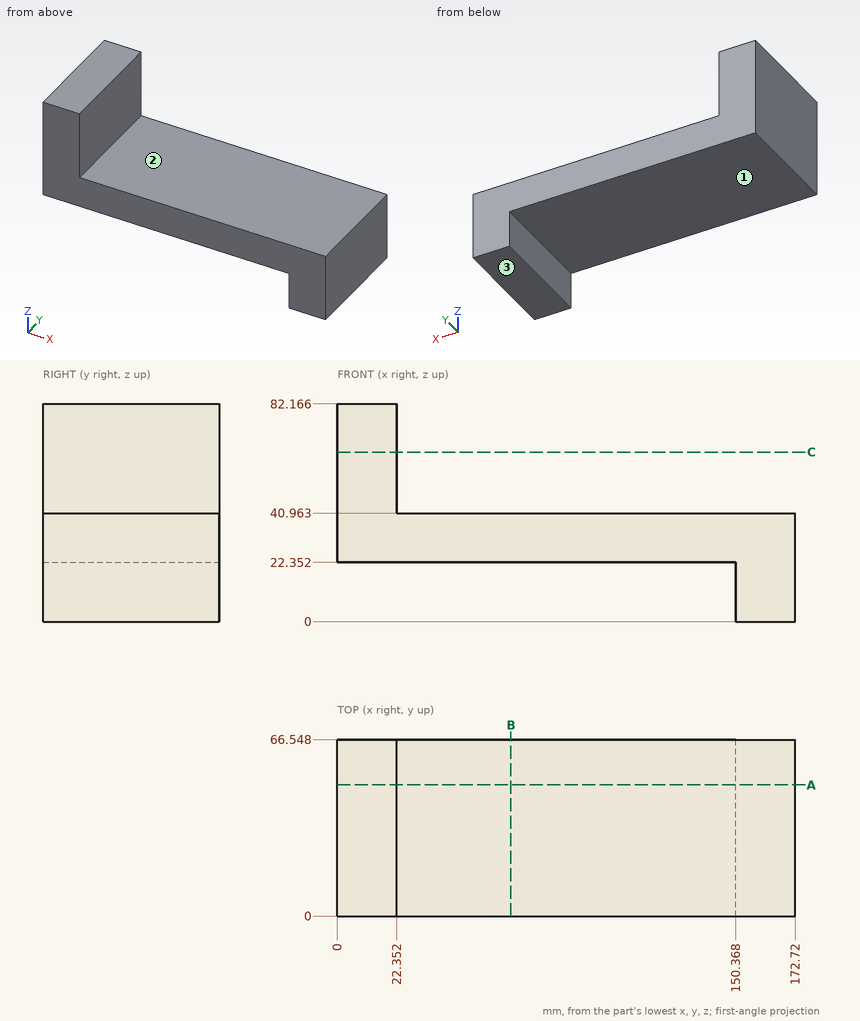
Verification items for this drawing (mm, ordinates from the low corner). A direction names the side the tool comes from. Coordinates: 2 decimals unless noted, no trailing zeros. Write each loop counter-clockwise with the first axis right and the second up, starting at its lowest first coordinate (ties: lowest second). Pieces come first, ordered by that corner, then holes. Notation, with made-up numbers: M 21.5,-36.5 L 72.5,-36.5 A4 cw 72.5,-31.5 Z; hole C 84.25,-34 d11. An arc over 180 degrees is marked long. Use CSV: the item, a comma, the result in double quotes.
Q1. Thickness scan on line 1 along Z through (x, y) = (90.5, 59); line 2 along X through (y, z) = (62, 21.5); line 3 along X through (y, z) = (21.5, 61). Record the ranges inside material, lowest first. Write a range as [from, to].
Computed values:
line 1,"[22.35, 40.96]"
line 2,"[150.37, 172.72]"
line 3,"[0, 22.35]"
Q2. Section check A-A, the plane y = 49.5. Enter the section's corners in (x, z) (1 decimal).
Computed values:
outline,"M 0,22.4 L 150.4,22.4 L 150.4,0 L 172.7,0 L 172.7,41 L 22.4,41 L 22.4,82.2 L 0,82.2 Z"
Q3. Set-up check for the marked faces 1, 2 and 3: record each of +Z, -Z, +X, -X, +Y, -Y from which the full face is reachable in a straight line by a thin tool's end or side.
Computed values:
face 1,"-Z, -X, +Y, -Y"
face 2,"+Z, +X, +Y, -Y"
face 3,"-Z, +X, -X, +Y, -Y"
Q4. Section check C-C, the plane z = 64. Enter the section's corners in (x, y).
Computed values:
outline,"M 0,0 L 22.35,0 L 22.35,66.55 L 0,66.55 Z"
Q5. Go/stop test with flat-tipped pins: P1, Ø6.5, axis at y = 29.5, z = 10, coming from the -X side; P2, Ø20, axis at x = 43.5, y = 38.5, coming from the -Z side; P3, Ø20.5, axis at y = 40, z = 52.5, coming from the +X side. Record where each tip stops, or that it passes through.
Computed values:
P1,"x = 150.37"
P2,"z = 22.35"
P3,"x = 22.35"
Q6. Section check B-B, the plane x = 65.5. Enter the section's corners in (y, z), and give its area (3 significant figures).
Computed values:
outline,"M 0,22.35 L 66.55,22.35 L 66.55,40.96 L 0,40.96 Z"
area,"1,240 mm²"
